from build123d import *

# Parameters (mm, degrees)
F0_W     = 184.4834834337
F0_H     = 71.9514358789
F1_DEPTH = 66.04
F2_T     = -5.08
F3_DEPTH = 33.02
F4_R     = 5.08
F5_R     = 5.08


with BuildPart() as f1:
    # F0 (on Front) → F1 (new body)
    with BuildSketch(Plane.XZ):
        with Locations((1.5829280019, 5.4683079943)):
            Rectangle(F0_W, F0_H)
    extrude(amount=F1_DEPTH)

    # F2
    f2_openings = [f1.faces().sort_by_distance(p)[0] for p in [
        (1.582928, -66.04, 5.468308),
    ]]
    offset(amount=F2_T, openings=f2_openings)

    # F3 (cut): a face of the model
    f3_faces = [f1.faces().sort_by_distance(p)[0] for p in [
        (1.5829280019, -5.08, 5.4683079943),
    ]]
    extrude(f3_faces, amount=F3_DEPTH, mode=Mode.SUBTRACT)

    # F4
    f4_edges = [f1.edges().sort_by_distance(p)[0] for p in [
        (-90.658814, -33.02, 41.444026),
        (93.82467, -33.02, 41.444026),
        (93.82467, -33.02, -30.50741),
        (-90.658814, -33.02, -30.50741),
    ]]
    fillet(f4_edges, radius=F4_R)

    # F5
    f5_edges = [f1.edges().sort_by_distance(p)[0] for p in [
        (-85.578814, -35.56, -25.42741),
        (88.74467, -35.56, -25.42741),
        (88.74467, -35.56, 36.364026),
        (-85.578814, -35.56, 36.364026),
    ]]
    fillet(f5_edges, radius=F5_R)


solid = f1.part
Work out the finished part from the listing and answer in its coordinate system (mm). A direction names the side the tool comes from. Round coordinates to 2 decimals unless told otherwise and drop trailing zeros. Loops run counter-clockwise (first coordinate to the right, second up) from the corner with the lowest first, then second, coordinate; pieces in that order, holes last. Notation, with made-up numbers: (34.25, 68.25) -> (52.25, 68.25) arc R6 ccw to (52.25, 74.25) -> close; hole circle Ø11 at (25, -29.75). An arc over 180 degrees is marked (long way). Use one line per item in the form item = value.
(1) Find section A-A on y = -60.5. Give the vertices of the cut face in (x, z).
Answer list:
outline = (-90.66, -25.43) arc R5.08 ccw to (-85.58, -30.51) -> (88.74, -30.51) arc R5.08 ccw to (93.82, -25.43) -> (93.82, 36.36) arc R5.08 ccw to (88.74, 41.44) -> (-85.58, 41.44) arc R5.08 ccw to (-90.66, 36.36) -> close; hole (-85.58, -20.35) arc R5.08 ccw to (-80.5, -25.43) -> (83.66, -25.43) arc R5.08 ccw to (88.74, -20.35) -> (88.74, 31.28) arc R5.08 ccw to (83.66, 36.36) -> (-80.5, 36.36) arc R5.08 ccw to (-85.58, 31.28) -> close
(2) Find section B-B on z = 28. Give the vertices of the cut face in (x, y), then the cut area to 3 significant figures.
Answer list:
outline = (-90.66, -66.04) -> (-85.58, -66.04) -> (-85.58, -5.08) -> (88.74, -5.08) -> (88.74, -66.04) -> (93.82, -66.04) -> (93.82, 0) -> (-90.66, 0) -> close
area = 1,560 mm2
(3) For a pull along X with two mould halves and no side action, classify faces 3 (the cylindrical face through (92.376, -33.482, 39.916)), 4 (the cylindrical face through (-89.21, -33.48, -28.98)), 5 (the cylindrical face through (-84.13, -35.987, 34.836)) as released by +X, released by -X, zero draft, split by the parting line, or undercut.
Answer list:
face_3 = released by +X
face_4 = released by -X
face_5 = undercut
(4) A flat-ended cylindrical pin translates along its axis: P1, Ø2, axis at x = -17, z = 13, coming from the -Y side. Find the tip coordinate at first contact, or state that the pin passes through.
Answer list:
P1 = -5.08
(5) Straight lines are drawn through the part: line 1 (Z direction, x = -28.5, y = -23.5); line 2 (X direction, y = -19, z = 3); line 3 (Y direction, x = 37, z = 31). For each, find the intervals that lie inside material, in ascending order.
Answer list:
line_1 = -30.51 to -25.43, 36.36 to 41.44
line_2 = -90.66 to -85.58, 88.74 to 93.82
line_3 = -5.08 to 0
(6) Find section C-C on x = 71.5. Give the vertices of the cut face in (y, z).
Answer list:
outline = (-66.04, -30.51) -> (0, -30.51) -> (0, 41.44) -> (-66.04, 41.44) -> (-66.04, 36.36) -> (-5.08, 36.36) -> (-5.08, -25.43) -> (-66.04, -25.43) -> close
(7) A tool of negligible diameter and unlimited length cuts with its end or side. For faces 1 (the cylindrical face through (92.376, -33.482, -28.98)), 2 (the flat face through (88.745, -35, 5)), from which of +Z, -Z, +X, -X, +Y, -Y can it reach the whole face along a straight path? Write none if from no direction.
Answer list:
face_1 = -Z, +X, +Y, -Y
face_2 = -Y
